Geometry check sheet. Reference: the model listing, model coordinates, mm. A direction names the side the tool comes from. Round coordinates to 2 decimals unless told otherwise and drop trailing zeros. Order: outer loops, then holes, each group sorted by start corner. A loop starts at its lowest first (then second) coordinate and runs counter-clockwise, first axis right, second up. Notation, with made-up numbers: (43, 38) -> (57, 38) arc R29 ccw to (57, 74) -> close; hole circle Ø1 at (-26, 78.5). An arc over 180 degrees is marked (long way). Use a Markdown table: item, result. Add a question column.
Item 1: Sectioned sample at B-B, the plane z = 0. Record the cut outline in (x, y), and give its area (3 significant figures).
Item 2: Sectioned sample at C-C, the plane y = 1.8. Record the cut outline in (x, z).
Item 3: Set-up check for faces 1 (the flat face through (0, 0, 4)), 2 (the flat face through (-1.3, 3.2, 1.3)): record each of +Z, -Z, +X, -X, +Y, -Y from which the full face is reachable in a straight line by a thin tool's end or side.
Item 4: Gauge pin test, flat ends, axial feed: pin 1 Ø3 at (x, y) = (3.5, 3.5) entering from +Z; pin 2 Ø1.5 at (x, y) = (-14.5, 1.5) entering from -Z; pin 3 Ø2 at (x, y) = (12, 2.5) entering from +Z. Record the tip position at first contact, or that the pin passes through.
Item 5: Mould release check, pull along Z, two halves, no side actions. Record for faces 3 (the cylindrical face through (-0.97, 1.62, -1.27)), 4 (the cylindrical face through (-19.524, 1.479, -4.336)), 5 (the flat face through (-4, 5, 0)): pulls with the +Z half, pulls with the -Z half, needs draft (parallel to the pull), parting line crosses it, or undercut.
Item 6: Sectioned sample at A-A, the plane x = 0. Record the cut outline in (y, z), and give its area (3 significant figures).
Item 7: Material ranges on probe 1 along X at (y, z) = (2.2, 0); probe 2 along X at (y, z) = (4.45, -2); probe 3 along Z at (x, y) = (10.5, 2.8), recorded low to high. Write a range as [from, to].
from build123d import *

# Parameters (mm, degrees)
SKETCH_1_R          = 20
EXTRUDE_1_DEPTH     = 5
FILLET_1_R          = 2
SKETCH_2_R          = 3
CUT_EXTRUDE_1_DEPTH = 1.8
SKETCH_3_R          = 1.6
CUT_EXTRUDE_2_DEPTH = 29.46471507


with BuildPart() as part:
    # 草图1 → 凸台-拉伸1 (new body)
    with BuildSketch(Plane(origin=(0, 0, 0), x_dir=(1, 0, 0), z_dir=(0, 1, 0))):
        with Locations(Location((0, 0, 0), (0, 0, 270))):
            Circle(SKETCH_1_R)
    extrude(amount=EXTRUDE_1_DEPTH)

    # 圆角1
    fillet_1_edges = [part.edges().sort_by_distance(p)[0] for p in [
        (0, 5, -20),
    ]]
    fillet(fillet_1_edges, radius=FILLET_1_R)

    # 草图2 → 切除-拉伸1 (cut)
    with BuildSketch(Plane(origin=(0, 5, 0), x_dir=(1, 0, 0), z_dir=(0, 1, 0))):
        with Locations(Location((0, 0, 0), (0, 0, 270))):
            Circle(SKETCH_2_R)
    extrude(amount=-CUT_EXTRUDE_1_DEPTH, mode=Mode.SUBTRACT)

    # 草图3 → 切除-拉伸2 (cut, through all)
    with BuildSketch(Plane(origin=(0, 3.2, 0), x_dir=(1, 0, 0), z_dir=(0, 1, 0))):
        with Locations(Location((0, 0, 0), (0, 0, 270))):
            Circle(SKETCH_3_R)
    extrude(amount=-CUT_EXTRUDE_2_DEPTH, mode=Mode.SUBTRACT)


solid = part.part
Found:
| question | item | result |
|---|---|---|
| 1 | outline | (-20, 0) -> (-1.6, 0) -> (-1.6, 3.2) -> (-3, 3.2) -> (-3, 5) -> (-18, 5) arc R2 ccw to (-20, 3) -> close; (1.6, 0) -> (20, 0) -> (20, 3) arc R2 ccw to (18, 5) -> (3, 5) -> (3, 3.2) -> (1.6, 3.2) -> close |
| 1 | area | 177 mm2 |
| 2 | outline | circle Ø40 at (0, 0); hole circle Ø3.2 at (0, 0) |
| 3 | face 1 | +Z, -Z, +X, -X, -Y |
| 3 | face 2 | +Y |
| 4 | pin 1 | stops at z = 19.89 |
| 4 | pin 2 | stops at z = -14.52 |
| 4 | pin 3 | stops at z = 16.7 |
| 5 | face 3 | undercut |
| 5 | face 4 | parting line crosses it |
| 5 | face 5 | needs draft |
| 6 | outline | (0, -20) -> (3, -20) arc R2 ccw to (5, -18) -> (5, -3) -> (3.2, -3) -> (3.2, -1.6) -> (0, -1.6) -> close; (0, 1.6) -> (3.2, 1.6) -> (3.2, 3) -> (5, 3) -> (5, 18) arc R2 ccw to (3, 20) -> (0, 20) -> close |
| 6 | area | 177 mm2 |
| 7 | probe 1 | x = [-20, -1.6], [1.6, 20] |
| 7 | probe 2 | x = [-19.27, -2.24], [2.24, 19.27] |
| 7 | probe 3 | z = [-17.02, 17.02] |
